```python
from build123d import *

# Parameters (mm, degrees)
CROQUIS1_W              = 57.2
CROQUIS1_H              = 10.7
SALIENTE_EXTRUIR1_DEPTH = 1.45
CROQUIS2_W              = 5
CROQUIS2_H              = 5
SALIENTE_EXTRUIR2_DEPTH = 1.55
MATRIZL1_COUNT          = 8
MATRIZL1_PITCH          = 7.1
CORTAR_EXTRUIR1_REACH   = 3.45
CROQUIS3_R              = 1.5
CROQUIS4_W              = 1.8
CROQUIS4_H              = 1
SALIENTE_EXTRUIR3_DEPTH = 0.8


with BuildPart() as part:
    # Croquis1 → Saliente-Extruir1 (new body)
    with BuildSketch(Plane.XY):
        with Locations((28.6, 5.35)):
            Rectangle(CROQUIS1_W, CROQUIS1_H)
    extrude(amount=SALIENTE_EXTRUIR1_DEPTH)

    # Croquis2 → Saliente-Extruir2 (add)
    with BuildSketch(Plane.XY.offset(1.45)):
        with Locations((3.9, 7.7)):
            Rectangle(CROQUIS2_W, CROQUIS2_H)
    saliente_extruir2 = extrude(amount=SALIENTE_EXTRUIR2_DEPTH)

    # MatrizL1: Saliente-Extruir2 ×8
    with Locations(*[(i * MATRIZL1_PITCH, 0, 0) for i in range(1, MATRIZL1_COUNT)]):
        add(saliente_extruir2)

    # Croquis3 → Cortar-Extruir1 (cut, up to next)
    with BuildSketch(Plane.XY.offset(1.45), mode=Mode.PRIVATE) as cortar_extruir1_sk1:
        with Locations((14.7, 2.3)):
            Circle(CROQUIS3_R)
    cortar_extruir1_tool1 = extrude(cortar_extruir1_sk1.sketch, amount=-CORTAR_EXTRUIR1_REACH, mode=Mode.PRIVATE) & part.part
    add(cortar_extruir1_tool1.solids().sort_by_distance((14.7, 2.3, 1.45))[0], mode=Mode.SUBTRACT)
    # Croquis3 → Cortar-Extruir1 (cut, up to next)
    with BuildSketch(Plane.XY.offset(1.45), mode=Mode.PRIVATE) as cortar_extruir1_sk2:
        with Locations((42.5, 2.3)):
            Circle(CROQUIS3_R)
    cortar_extruir1_tool2 = extrude(cortar_extruir1_sk2.sketch, amount=-CORTAR_EXTRUIR1_REACH, mode=Mode.PRIVATE) & part.part
    add(cortar_extruir1_tool2.solids().sort_by_distance((42.5, 2.3, 1.45))[0], mode=Mode.SUBTRACT)

    # Croquis4 → Saliente-Extruir3 (add)
    with BuildSketch(Plane.XY.offset(1.45)):
        with Locations((3.1, 1.5)):
            Rectangle(CROQUIS4_W, CROQUIS4_H)
        with Locations((8.6, 1.5)):
            Rectangle(CROQUIS4_W, CROQUIS4_H)
        with Locations((20.3, 1.5)):
            Rectangle(CROQUIS4_W, CROQUIS4_H)
        with Locations((25.4, 1.5)):
            Rectangle(CROQUIS4_W, CROQUIS4_H)
        with Locations((31.5, 1.5)):
            Rectangle(CROQUIS4_W, CROQUIS4_H)
        with Locations((36.6, 1.5)):
            Rectangle(CROQUIS4_W, CROQUIS4_H)
        with Locations((48.3, 1.5)):
            Rectangle(CROQUIS4_W, CROQUIS4_H)
        with Locations((54.1, 1.5)):
            Rectangle(CROQUIS4_W, CROQUIS4_H)
    extrude(amount=SALIENTE_EXTRUIR3_DEPTH)


solid = part.part
```
The model under review builds one solid part; all positions refer to its coordinate system, in mm. A direction names the side the tool comes from. Give positions to 0.01 mm unless a question says otherwise; leave off trailing zeros. Write each loop counter-clockwise with the first axis right and the second up, starting at its lowest first coordinate (ties: lowest second). Pieces come first, ordered by that corner, then holes. Notation, with made-up numbers: M 20,82.5 L 25,82.5 A17 cw 25,103.5 Z; hole C 30.5,33.25 d10. An arc over 180 degrees is marked long. Write item = value, one per line. Start each with the question number.
Q1. Machinability: for faces 5 (the face through (20.3, 1.5, 2.25)), 6 (the face through (11, 10.2, 2)), 7 (the face through (32, 5.2, 2)), which of the approach directions +Z, -Z, +X, -X, +Y, -Y give a long, thin tool a straight path to every point of the face, cutting with its end or side? Answer none if there is none.
Q2. We need section B-B (x = 9). State the section outline as (y, z) points, plus the area to 3 significant figures.
Q3. We need section A-A (x = 42.5). State the section outline as (y, z) points.
Q4. For line 1 (Y direction, x = 14.7, z = 0.75); line 2 (Z direction, x = 7, y = 10.25); line 3 (Y direction, x = 12, z = 1.95), list the stretches that pass through material, from the lowest coordinate up.
Q5. Mouldability with a two-part tool opening along X and no side actions: class faces 1 (the face through (57.2, 5, 1)), 2 (the face through (20.6, 8, 2)), 3 (the face through (36.9, 8, 2)), 4 (the face through (39, 10.2, 2)) as released by +X, released by -X, zero draft, split by the parting line, or undercut.
Q6. Clearance check with flat-ended pins moving along their axes: pin 1 (0.8 mm diameter, centred on x = 38, z = 2.5, fed in from -Y); pin 2 (0.6 mm diameter, centred on y = 1.5, z = 2, fed in from -X); pin 3 (0.5 mm diameter, centred on x = 46, z = 2, fed in from +Y). State where each tip first meets the part, or that it passes through.
Result set:
q1.face_5 = +Z, +X, -X, -Y
q1.face_6 = +Z, +X, -X, +Y
q1.face_7 = +Z, +X, -X
q2.outline = M 0,0 L 10.7,0 L 10.7,1.45 L 10.2,1.45 L 10.2,3 L 5.2,3 L 5.2,1.45 L 2,1.45 L 2,2.25 L 1,2.25 L 1,1.45 L 0,1.45 Z
q2.area = 24.1 mm2
q3.outline = M 0,0 L 0.8,0 L 0.8,1.45 L 0,1.45 Z; M 3.8,0 L 10.7,0 L 10.7,1.45 L 3.8,1.45 Z
q4.line_1 = 0 to 0.8, 3.8 to 10.7
q4.line_2 = 0 to 1.45
q4.line_3 = 5.2 to 10.2
q5.face_1 = released by +X
q5.face_2 = undercut
q5.face_3 = undercut
q5.face_4 = zero draft
q6.pin_1 = 5.2
q6.pin_2 = 2.2
q6.pin_3 = 10.2
